CAD build for the part. Positions are in the model's coordinates, mm. A direction names the side the tool comes from. Round coordinates to 2 decimals unless told otherwise and drop trailing zeros. Order: outer loops, then holes, each group sorted by start corner. A loop starts at its lowest first (then second) coordinate and runs counter-clockwise, first axis right, second up. Notation, with made-up numbers: M 20,42 L 40,42 A18 ccw 40,67 Z; hole C 87.5,-17 d4. An arc over 180 degrees is marked long. Answer as a JSON object with one key per item and string values.
```python
from build123d import *

# Parameters (mm, degrees)
SKETCH1_W           = 100
SKETCH1_H           = 70
SKETCH1_R           = 1.5
SKETCH1_R_2         = 2.5
BOSS_EXTRUDE1_DEPTH = 2
SKETCH2_W           = 70
SKETCH2_H           = 2
BOSS_EXTRUDE2_DEPTH = 70
SKETCH3_W           = 70
SKETCH3_H           = 2
BOSS_EXTRUDE3_DEPTH = 4.57
SKETCH4_W           = 34.57
SKETCH4_H           = 2
BOSS_EXTRUDE4_DEPTH = 70
SKETCH5_R           = 2
CUT_EXTRUDE1_DEPTH  = 10


with BuildPart() as part:
    # Sketch1 → Boss-Extrude1 (new body)
    with BuildSketch(Plane(origin=(0, 0, 0), x_dir=(1, 0, 0), z_dir=(0, 1, 0))):
        Rectangle(SKETCH1_W, SKETCH1_H)
        with Locations((25.755, 20.98)):
            Circle(SKETCH1_R, mode=Mode.SUBTRACT)
        with Locations((-25.755, 20.98)):
            Circle(SKETCH1_R, mode=Mode.SUBTRACT)
        with Locations((25.755, -20.52)):
            Circle(SKETCH1_R, mode=Mode.SUBTRACT)
        with Locations((-25.755, -20.52)):
            Circle(SKETCH1_R, mode=Mode.SUBTRACT)
        with Locations((-25.755, -0.05)):
            Circle(SKETCH1_R_2, mode=Mode.SUBTRACT)
    extrude(amount=BOSS_EXTRUDE1_DEPTH)

    # Sketch2 → Boss-Extrude2 (add)
    with BuildSketch(Plane(origin=(0, 2, 0), x_dir=(1, 0, 0), z_dir=(0, 1, 0))):
        with Locations((-15, -36)):
            Rectangle(SKETCH2_W, SKETCH2_H)
    extrude(amount=-BOSS_EXTRUDE2_DEPTH)

    # Sketch3 → Boss-Extrude3 (add)
    with BuildSketch(Plane(origin=(50, 0, 0), x_dir=(0, 0, -1), z_dir=(1, 0, 0))):
        with Locations((0, 1)):
            Rectangle(SKETCH3_W, SKETCH3_H)
    extrude(amount=BOSS_EXTRUDE3_DEPTH)

    # Sketch4 → Boss-Extrude4 (add)
    with BuildSketch(Plane(origin=(0, 2, 0), x_dir=(1, 0, 0), z_dir=(0, 1, 0))):
        with Locations((37.285, -36)):
            Rectangle(SKETCH4_W, SKETCH4_H)
    extrude(amount=-BOSS_EXTRUDE4_DEPTH)

    # Sketch5 → Cut-Extrude1 (cut)
    with BuildSketch(Plane(origin=(0, 0, 35), x_dir=(-1, 0, 0), z_dir=(0, 0, -1))):
        with Locations((-32.285, -18)):
            Circle(SKETCH5_R)
        with Locations((27.715, -48)):
            Circle(SKETCH5_R)
        with Locations((-32.285, -48)):
            Circle(SKETCH5_R)
        with Locations((27.715, -18)):
            Circle(SKETCH5_R)
    extrude(amount=-CUT_EXTRUDE1_DEPTH, mode=Mode.SUBTRACT)


solid = part.part
```
Item 1: Wall check: line 1 along Y through (x, z) = (27.5, -13.5); line 2 along Z through (x, y) = (-45, -0.5). Give the ranges that are in metal, low to high. Write a range as [from, to].
Worked answers:
{"line 1": "y = [0, 2]", "line 2": "z = [35, 37]"}
Item 2: Two-plate mould, pull along X, no slides. Class faces 1 (the flat face through (54.57, 1, 17)), 2 (the flat face through (2, 2, 0)), 3 (the flat face through (-50, 1, 17)), 4 (the cylindrical face through (-24.369, 0.986, 21.095)): released by +X, released by -X, zero draft, split by the parting line, or undercut.
Worked answers:
{"face 1": "released by +X", "face 2": "zero draft", "face 3": "released by -X", "face 4": "undercut"}
Item 3: Saw through at C-C on z = 20.52. List the corners of the cut face in (x, y) (3 decimals), and give its area (3 significant figures).
Worked answers:
{"outline": "M -50,0 L -27.255,0 L -27.255,2 L -50,2 Z; M -24.255,0 L 24.255,0 L 24.255,2 L -24.255,2 Z; M 27.255,0 L 54.57,0 L 54.57,2 L 27.255,2 Z", "area": "197 mm2"}
Item 4: Drop flat-ended pins along their axis: pin 1 Ø3.5 at (x, y) = (32.285, -48) entering from +Z; pin 2 Ø2 at (x, z) = (35.5, -21.5) entering from -Y; pin 3 Ø4 at (x, y) = (6, -23.5) entering from -Z. Give the stop position or say it passes through.
Worked answers:
{"pin 1": "passes through", "pin 2": "stops at y = 0", "pin 3": "stops at z = 35"}
Item 5: 3-axis set-ups, long thin cutter, end or side, ignore diameter. For faces 5 (the flat face through (2, -34, 35)), 6 (the cylindrical face through (-27.455, -16.017, 35.986)): which of +Z, -Z, +X, -X, +Y, -Y reach the whole face in a straight line?
Worked answers:
{"face 5": "-Z, +X, -X, -Y", "face 6": "+Z, -Z"}
Item 6: Saw through at A-A on z = 0.05. List the corners of the cut face in (x, y) (3 decimals), and give its area (3 significant figures).
Worked answers:
{"outline": "M -50,0 L -28.255,0 L -28.255,2 L -50,2 Z; M -23.255,0 L 54.57,0 L 54.57,2 L -23.255,2 Z", "area": "199 mm2"}
Item 7: Saw through at B-B on y = -48. List the corners of the cut face in (x, z) (3 decimals).
Worked answers:
{"outline": "M -50,35 L -29.715,35 L -29.715,37 L -50,37 Z; M -25.715,35 L 30.285,35 L 30.285,37 L -25.715,37 Z; M 34.285,35 L 54.57,35 L 54.57,37 L 34.285,37 Z"}
Item 8: Saw through at D-D on x = -37.5. List the corners of the cut face in (y, z).
Worked answers:
{"outline": "M -68,35 L 0,35 L 0,-35 L 2,-35 L 2,37 L -68,37 Z"}
